from build123d import *

# Parameters (mm, degrees)
SKETCH1_R             = 20
BOSS_EXTRUDE1_DEPTH   = 40
SKETCH2_W             = 50
SKETCH2_H             = 40
BOSS_EXTRUDE2_DEPTH   = 5
BOSS_EXTRUDE2_2_DEPTH = 5
SKETCH7_R             = 2
BOSS_EXTRUDE3_DEPTH   = 50
SKETCH9_R             = 4.5
SKETCH9_R_2           = 2.15
CUT_EXTRUDE1_DEPTH    = 30
SKETCH9_3_R           = 2.15
CUT_EXTRUDE2_DEPTH    = 88.321246052


with BuildPart() as part:
    # Sketch1 → Boss-Extrude1 (new body)
    with BuildSketch(Plane(origin=(0, 0, 0), x_dir=(1, 0, 0), z_dir=(0, 1, 0))):
        with Locations(Location((0, 0, 0), (0, 0, 270))):
            Circle(SKETCH1_R)
    extrude(amount=BOSS_EXTRUDE1_DEPTH)



with BuildPart() as body_2:
    # Sketch2 → Boss-Extrude2 (new, symmetric)
    with BuildSketch(Plane.XY):
        with Locations((50, 20)):
            Rectangle(SKETCH2_W, SKETCH2_H)
    extrude(amount=BOSS_EXTRUDE2_DEPTH, both=True)


with BuildPart() as body_3:
    # Sketch2 → Boss-Extrude2 2 (new, symmetric)
    with BuildSketch(Plane.XY):
        with Locations((-50, 20)):
            Rectangle(SKETCH2_W, SKETCH2_H)
    extrude(amount=BOSS_EXTRUDE2_2_DEPTH, both=True)


with BuildPart() as part_1:
    add(part.part)

    add(body_2.part)  # Boss-Extrude3 merges body 2

    add(body_3.part)  # Boss-Extrude3 merges body 3
    # Sketch7 → Boss-Extrude3 (add, symmetric)
    with BuildSketch(Plane(origin=(0, 0, 0), x_dir=(0, 0, -1), z_dir=(1, 0, 0))):
        with Locations(Location((0, 20, 0), (0, 0, 180))):
            Circle(SKETCH7_R)
    extrude(amount=BOSS_EXTRUDE3_DEPTH, both=True)

    # Sketch9 → Cut-Extrude1 (cut)
    # profile 1 of 2: a face of its own
    with BuildSketch(Plane(origin=(0, 40, 0), x_dir=(1, 0, 0), z_dir=(0, 1, 0))):
        with Locations(Location((0, 0, 0), (0, 0, 270))):
            Circle(SKETCH9_R)
        Circle(SKETCH9_R_2, mode=Mode.SUBTRACT)
    # profile 2 of 2: a face of its own
    with BuildSketch(Plane(origin=(0, 40, 0), x_dir=(1, 0, 0), z_dir=(0, 1, 0))):
        Circle(SKETCH9_R_2)
    extrude(amount=-CUT_EXTRUDE1_DEPTH, mode=Mode.SUBTRACT)

    # Sketch9_3 → Cut-Extrude2 (cut, through all)
    with BuildSketch(Plane(origin=(0, 40, 0), x_dir=(1, 0, 0), z_dir=(0, 1, 0))):
        with Locations(Location((0, 0, 0), (0, 0, 270))):
            Circle(SKETCH9_3_R)
    extrude(amount=-CUT_EXTRUDE2_DEPTH, mode=Mode.SUBTRACT)


solid = part_1.part
Build history of the part. All positions in model axes, mm. A direction names the side the tool comes from. Give positions to 0.01 mm unless a question says otherwise; leave off trailing zeros. Loops run counter-clockwise (first coordinate to the right, second up) from the corner with the lowest first, then second, coordinate; pieces in that order, holes last. Notation, with made-up numbers: (59, 11) -> (80, 11) arc R16 cw to (80, 41) -> close; hole circle Ø1 at (88, 4.5). An arc over 180 degrees is marked (long way). Answer in a Markdown table with one row per item.
Item 1: Slice it at D-D on x = 33. Write the cut outline in (y, z).
Findings below:
| item | result |
|---|---|
| outline | (0, -5) -> (40, -5) -> (40, 5) -> (0, 5) -> close |
Item 2: Slice it at A-A on y = 15. Write the cut outline in (x, z).
Findings below:
| item | result |
|---|---|
| outline | (-75, -5) -> (-25, -5) -> (-25, 5) -> (-75, 5) -> close; circle Ø40 at (0, 0); (25, -5) -> (75, -5) -> (75, 5) -> (25, 5) -> close; hole circle Ø9 at (0, 0) |
Item 3: Slice it at C-C on z = -9.5. Write the cut outline in (x, y), plus the area to 3 significant figures.
Findings below:
| item | result |
|---|---|
| outline | (-17.6, 0) -> (17.6, 0) -> (17.6, 40) -> (-17.6, 40) -> close |
| area | 1,410 mm² |
Item 4: Flat gauge pins, fed straight in: P1, Ø7, axis at x = 0, z = 0, coming from the -Y side; P2, Ø6, axis at x = 20, y = 6.5, coming from the +Z side; P3, Ø2, axis at x = 3, y = 32, coming from the -Z side; P4, Ø20, axis at x = -49.5, y = 20, coming from the -Z side. Where does each tip first touch, or does it go through?
Findings below:
| item | result |
|---|---|
| P1 | stops at y = 0 |
| P2 | stops at z = 10.54 |
| P3 | stops at z = -19.9 |
| P4 | stops at z = -5 |
Item 5: Mould opens along Z. For faces 1 (the flat face through (-50, 20, -5)), 2 (the flat face through (75, 20, 0)), 3 (the flat face through (-50, 20, 5)), 4 (the cylindrical face through (-1.308, 5.07, -1.706)) say: pulls with the +Z half, pulls with the -Z half, needs draft (parallel to the pull), parting line crosses it, or undercut.
Findings below:
| item | result |
|---|---|
| face 1 | pulls with the -Z half |
| face 2 | needs draft |
| face 3 | pulls with the +Z half |
| face 4 | undercut |
Item 6: Probe line 1 along X through (y, z) = (3.25, 0); line 2 along X through (y, z) = (6.5, 1); line 3 along X through (y, z) = (20.25, 0). List the from-to ranges inside material, lowest first. Write a range as [from, to].
Findings below:
| item | result |
|---|---|
| line 1 | x = [-75, -25], [-20, -2.15], [2.15, 20], [25, 75] |
| line 2 | x = [-75, -25], [-19.97, -1.9], [1.9, 19.97], [25, 75] |
| line 3 | x = [-75, -4.5], [4.5, 75] |
Item 7: Tool access for faces 5 (the flat face through (50, 20, 5)), 6 (the flat face through (5, 40, 0)), 7 (the cylindrical face through (1.352, 25.21, 4.292)), 8 (the flat face through (50, 20, -5)), 9 (the cylindrical face through (-22, 18, 0)): list every direction of +Z, -Z, +X, -X, +Y, -Y with a clear straight run to the whole face (end or side of a thin tool).
Findings below:
| item | result |
|---|---|
| face 5 | +Z, +X, +Y, -Y |
| face 6 | +Z, -Z, +X, -X, +Y |
| face 7 | +Y |
| face 8 | -Z, +X, +Y, -Y |
| face 9 | none |
Item 8: Slice it at B-B on x = 0. Write the cut outline in (y, z), plus the area to 3 significant figures.
Findings below:
| item | result |
|---|---|
| outline | (0, -20) -> (40, -20) -> (40, -4.5) -> (10, -4.5) -> (10, -2.15) -> (0, -2.15) -> close; (0, 2.15) -> (10, 2.15) -> (10, 4.5) -> (40, 4.5) -> (40, 20) -> (0, 20) -> close |
| area | 1,290 mm² |
